```python
from build123d import *

# Parameters (mm, degrees)
F0_W     = 50
F0_H     = 20.75
F3_DEPTH = 50.001
F4_COUNT = 9


with BuildPart() as f1:
    # F0 (on Front) → F1 (revolve)
    with BuildSketch(Plane.XZ):
        with Locations((-25, 19.875)):
            Rectangle(F0_W, F0_H)
    revolve(axis=Axis((-20.0732499361, 0, 0), (1, 0, 0)))

    # F2 (on face) → F3 (cut, through all)
    with BuildSketch(Plane.YZ):
        with BuildLine():
            ThreePointArc((-8.6240252272, 15.9361409658), (-6.1974049971, 17.0272302886), (-3.6371673564, 17.7512087932))
            ThreePointArc((-3.6371673564, 17.7512087932), (-3.4777696522, 23.9342534629), (-3, 30.1008720804))
            ThreePointArc((-3, 30.1008720804), (-10.3461093356, 28.4257017788), (-17.0503342847, 24.9869686193))
            ThreePointArc((-17.0503342847, 24.9869686193), (-12.7205154565, 20.5701691072), (-8.6240252272, 15.9361409658))
        make_face()
    f3 = extrude(amount=-F3_DEPTH, mode=Mode.SUBTRACT)

    # F4: F3 ×9 about axis
    f4_axis = Axis((-20.0732499361, 0, 0), (1, 0, 0))
    for i in range(1, F4_COUNT):
        add(f3.rotate(f4_axis, i * 360 / F4_COUNT), mode=Mode.SUBTRACT)

    # F6 (on offset) → F7 (revolve, cut)
    with BuildSketch(Plane.YZ.offset(-23)):
        Polygon((-4.5322137317, 19.7616658885), (-6.8814452837, 18.9066155302), (-2.7772035638, 7.6303040808), (-0.4279720118, 8.4853544391), align=None)
    revolve(axis=Axis((-23, -3.7938283898, 10.4234578343), (0, 0.3420201433, -0.9396926208)), mode=Mode.SUBTRACT)


solid = f1.part
```
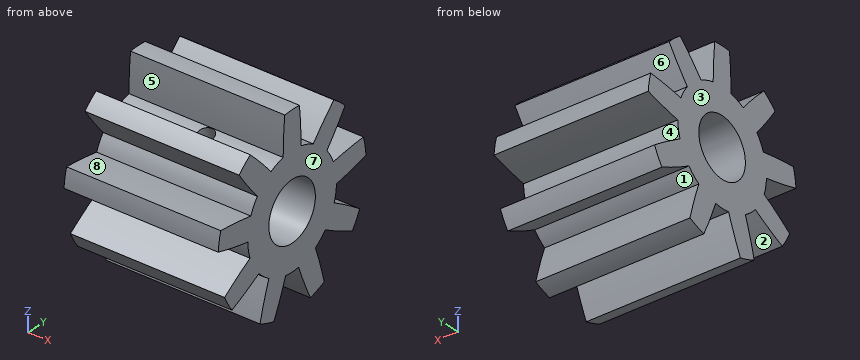
Geometry check sheet. Reference: the model listing, model coordinates, mm. Face numbers are marked on the shaded views. A direction names the side the tool comes from. Coordinates: 2 decimals unless noted, no trailing zeros. Loops run counter-clockwise (first coordinate to the right, second up) from the corner with the lowest first, then second, coordinate; pieces in that order, holes last.
Item 1: Sectioned sample at C-C, the plane z = -2.5. Record the boundary of the cut face in (x, y).
Item 2: Sectioned sample at A-A, the plane z = 23. Record the boundary of the cut face in (x, y), then the cut area to 3 significant figures.
Item 3: Access from +Z, -Z, +X, -X, +Y, -Y to the whole of each face (thin tool, end or side, straight path). Record for the marked faces 1, 2, 3, 4 and 5.
Item 4: Go/stop test with flat-tipped pins: pin 1 Ø12 at (x, y) = (-5.5, 16) entering from +Z; pin 2 Ø3 at (x, z) = (-10, 4.5) entering from +Y; pin 3 Ø5 at (x, z) = (-8, -8.5) entering from +Y. Record where each tip stops, or that it passes through.
Item 5: Release check for a two-part mould opening along Y. For the marked faces 6, 7 and 8 record: released by +Y, released by -Y, zero draft, split by the parting line, or undercut.
Item 6: Sectioned sample at B-B, the plane y = -16. Record the boundary of the cut face in (x, z), then the cut area to 3 significant figures.
Item 7: Thickness scan on line 1 (Y direction, x = -37.5, z = 23); line 2 (Z direction, x = -40.5, y = -21.5); line 3 (Z direction, x = -13, y = -16.5). Record the ranges inside material, lowest first.
Item 8: Sectioned sample at D-D, the plane z = -11. Record the boundary of the cut face in (x, y), then the cut area to 3 significant figures.
Check result:
1. outline: (-50, -17.95) - (0, -17.95) - (0, -9.17) - (-50, -9.17) - close; (-50, 9.17) - (0, 9.17) - (0, 17.95) - (-50, 17.95) - close
2. outline: (-50, -19.65) - (0, -19.65) - (0, -15.05) - (-50, -15.05) - close; (-50, -3.52) - (0, -3.52) - (0, 3.52) - (-50, 3.52) - close; (-50, 15.05) - (0, 15.05) - (0, 19.65) - (-50, 19.65) - close
2. area: 812 mm2
3. face 1: +X, -X
3. face 2: -Z, +X, -X
3. face 3: +Z, -Z, -X, +Y, -Y
3. face 4: +X, -X, +Y
3. face 5: +Z, +X, -X
4. pin 1: stops at z = 24.99
4. pin 2: stops at y = 30.1
4. pin 3: stops at y = 25.52
5. face 6: released by +Y
5. face 7: zero draft
5. face 8: undercut
6. outline: (-50, -13.4) - (0, -13.4) - (0, 8.5) - (-50, 8.5) - close; (-50, 13.46) - (0, 13.46) - (0, 23.96) - (-50, 23.96) - close
6. area: 1,620 mm2
7. line 1: y = -19.65 to -15.05, -3.52 to 3.52, 15.05 to 19.65
7. line 2: z = -16.22 to -8.34, 0.15 to 7.39, 20.91 to 21.28
7. line 3: z = -13.67 to 7.49, 14.09 to 24.45
8. outline: (-50, -25.52) - (0, -25.52) - (0, 25.52) - (-50, 25.52) - close
8. area: 2,550 mm2
